Autodesk Inventor part; units mm, degrees
ref_plane "YZ Plane" through (0, 0, 0) normal (1, 0, 0) x (0, 1, 0)
ref_plane "XZ Plane" through (0, 0, 0) normal (0, 1, 0) x (-1, 0, 0)
ref_plane "XY Plane" through (0, 0, 0) normal (0, 0, 1) x (1, 0, 0)
sketch "Sketch1" plane through (0, 0, 0) normal (1, 0, 0) x (0, 1, 0)
  line L0 (0, 0) -> (2.5, 0)
  line L1 (0, 0) -> (4, 0)
  line L2 (2.5, 0) -> (2.5, -7)
  line L3 (2.5, -7) -> (0, -7)
  line L4 (0, -7) -> (20, -7)
  line L5 (4, 0) -> (4, -7)
  line L6 (2.5, -7) -> (2.5, -41)
  line L7 (20, -7) -> (20, -11)
  line L8 (20, -11) -> (2.5, -11)
  line L9 (20, -7) -> (22.5, -7)
  line L10 (22.5, -7) -> (22.5, -11)
  line L11 (22.5, -11) -> (20, -11)
  line L12 (20, -11) -> (20, -7)
  line L13 (20, -7) -> (20, -11)
  line L14 (4, 0) -> (2.5, 0)
  line L15 (2.5, 0) -> (2.5, -11)
  line L16 (2.5, -11) -> (4, -11)
  line L17 (4, -11) -> (4, 0)
  line L18 (2.5, -11) -> (22.5, -11)
  line L19 (22.5, -11) -> (22.5, -7)
  line L20 (22.5, -7) -> (2.5, -7)
  line L21 (2.5, -7) -> (2.5, -11)
  line L22 (2.5, -11) -> (6.5, -11)
  line L23 (0, -7) -> (0, -105.9451)
  line L24 (2.5, -41) -> (25, -41)
  line L25 (0, -82) -> (2.5, -82)
  line L26 (0, -82) -> (4, -82)
  line L27 (2.5, -82) -> (2.5, -75)
  line L28 (2.5, -75) -> (0, -75)
  line L29 (0, -75) -> (20, -75)
  line L30 (4, -82) -> (4, -75)
  line L31 (20, -75) -> (20, -71)
  line L32 (20, -71) -> (2.5, -71)
  line L33 (20, -75) -> (22.5, -75)
  line L34 (22.5, -75) -> (22.5, -71)
  line L35 (22.5, -71) -> (20, -71)
  line L36 (20, -71) -> (20, -75)
  line L37 (20, -75) -> (20, -71)
  line L38 (4, -82) -> (2.5, -82)
  line L39 (2.5, -82) -> (2.5, -71)
  line L40 (2.5, -71) -> (4, -71)
  line L41 (4, -71) -> (4, -82)
  line L42 (2.5, -71) -> (22.5, -71)
  line L43 (22.5, -71) -> (22.5, -75)
  line L44 (22.5, -75) -> (2.5, -75)
  line L45 (2.5, -75) -> (2.5, -71)
  line L46 (2.5, -71) -> (6.5, -71)
  line L47 (2.5, -11) -> (6.5, -11)
  line L48 (6.5, -11) -> (6.5, -71)
  line L49 (6.5, -71) -> (2.5, -71)
  line L50 (2.5, -71) -> (2.5, -11)
  line L51 (6.5, -11) -> (9.5, -11)
  line L52 (9.5, -11) -> (9.5, -14)
  line L53 (9.5, -14) -> (6.5, -14)
  line L54 (6.5, -14) -> (6.5, -11)
  line L55 (6.5, -71) -> (9.5, -71)
  line L56 (9.5, -71) -> (9.5, -68)
  line L57 (9.5, -68) -> (6.5, -68)
  line L58 (6.5, -68) -> (6.5, -71)
  dimension "d1" = 2.5
  dimension "d2" = 4
  dimension "d3" = 7
  dimension "d4" = 20
  dimension "d5" = 34
  dimension "d9" = 4
  dimension "d12" = 2.5
  dimension "d13" = 4
  dimension "d55" = 22.5
  dimension "d56" = 4
  dimension "d80" = 3
  dimension "d81" = 3
  dimension "d82" = 3
  dimension "d83" = 3
revolve "Revolution2" add sketch "Sketch1" angle 360 about axis through (0, 0, -7) along (0, 0, -1) contours L1 L5 L4 L2 | L4 L17 L8 L6 | L4 L7 L8 L17 | L8 L48 L24 L6 | L9 L10 L11 L7 | L24 L48 L32 L50 | L8 L52 L53 L48 | L29 L30 L26 L27 | L39 L32 L41 L29 | L41 L32 L31 L29 | L57 L56 L32 L48 | L31 L35 L34 L33
sketch "Sketch6" plane through (0, 0, 0) normal (0, 1, 0) x (-1, 0, 0)
  line L0 (-2.5, -82) -> (2.5, -82)
  line L1 (0, -82) -> (0, -62)
  line L2 (0, -82) -> (20, -82) construction
  line L3 (0, -65) -> (15, -65) construction
  line L4 (0, -59) -> (15, -59) construction
  line L5 (10.6066, -48.3934) -> (10.6066, -54.3934)
  line L6 (0, -65) -> (0, -59)
  line L7 (0, -62) -> (0, -59.5)
  line L8 (0, -59.5) -> (10.6066, -48.8934)
  line L9 (10.6066, -48.8934) -> (10.6066, -53.8934)
  line L10 (10.6066, -53.8934) -> (0, -64.5)
  line L11 (0, -59.5) -> (0, -64.5)
  point P0 (0, 0)
  dimension "d64" = 20
  dimension "d65" = 90
  dimension "d69" = 15
  dimension "d71" = 15
  dimension "d75" = 2.5
  dimension "d76" = 5
extrude "Extrusion6" cut sketch "Sketch6" along normal mid plane 5
sketch "Sketch7" plane through (0, 0, 0) normal (0, 0, 1) x (1, 0, 0)
  arc A0 (-1.9966, -1.5104) -> (-1.9966, 1.4896) centre (0.0034, -0.0104) ccw
  line L0 (-1.9966, -0.0104) -> (-1.9966, 1.4896)
  line L1 (-1.9966, -0.0104) -> (-1.9966, -1.5104)
  line L2 (-1.9966, 1.4896) -> (-1.9966, -2.007)
  line L3 (-1.9966, -2.007) -> (-3.9862, -2.007)
  line L4 (-3.9862, -2.007) -> (-3.9862, 1.4896)
  line L5 (-3.9862, 1.4896) -> (-1.9966, 1.4896)
  line L6 (-1.9966, -1.5104) -> (-3.2272, -1.5104)
  line L7 (-3.2272, -1.5104) -> (-3.2272, 1.4896)
  line L8 (-3.2272, 1.4896) -> (-1.9966, 1.4896)
  line L9 (-1.9966, 1.4896) -> (-1.9966, -1.5104)
  point P0 (0, 0)
  point P1 (0, 0)
  dimension "d77" = 5
extrude "Extrusion7" add sketch "Sketch7" against normal blind 26 contours L6 L7 L5 L0 L1
sketch "Sketch11" plane through (0, 0, -71) normal (0, 0, 1) x (1, 0, 0)
  circle A0 centre (0, 0) radius 2.5
  circle A1 centre (0, 0) radius 9.5
  arc A2 (0, 2.5) -> (0, -2.5) centre (0, 0) ccw
  circle A3 centre (0, 0) radius 46.837
  point P0 (0, 0)
  dimension "d90" = 19
extrude "Extrusion11" cut sketch "Sketch11" against normal blind 100 contours A0 | A1 | A3
sketch "Sketch12" plane through (0, 0, -71) normal (0, 0, -1) x (-1, 0, 0)
  circle A0 centre (0, 0) radius 9.5
  circle A1 centre (0, 0) radius 9.5
  circle A2 centre (0, 0) radius 6.5
  point P0 (0, 0)
extrude "Extrusion12" add sketch "Sketch12" along normal blind 2
sketch "Sketch13" plane through (0, 0, -11) normal (0, 0, -1) x (-1, 0, 0)
  circle A0 centre (0, 0) radius 46.586
extrude "Extrusion13" cut sketch "Sketch13" against normal blind 30
sketch "Sketch14" plane through (0, 0, -11) normal (0, 0, 1) x (1, 0, 0)
  circle A0 centre (0, 0) radius 9.5
  circle A1 centre (0, 0) radius 9.5
  arc A2 (0, 2.5) -> (0, -2.5) centre (0, 0) ccw
  circle A3 centre (0, 0) radius 6.5
  dimension "d97" = 19
  dimension "d98" = 13
extrude "Extrusion14" add sketch "Sketch14" along normal blind 2
properties part number "Spool_revB3"
Read the model definition and answer for the solid it produces. Units are mm, in the model's axes. A direction names the side the tool comes from. Coordinates: 2 decimals unless noted, no trailing zeros. Write each loop counter-clockwise with the first axis right and the second up, starting at its lowest first coordinate (ties: lowest second). Pieces come first, ordered by that corner, then holes. Notation, with made-up numbers: M -38,-25 L -3,-25 A33 cw -3,14 Z; hole C 27,87 d3. An arc over 180 degrees is marked long. Use a Markdown table: item, result.
Q1. The part is cut by section A-A, the plane y = -7.5. Write down the section's boundary in (x, z).
Answer block:
| item | result |
|---|---|
| outline | M -5.83,-73 L 5.83,-73 L 5.83,-68 L -5.83,-68 Z; M -5.83,-14 L 5.83,-14 L 5.83,-9 L -5.83,-9 Z |
Q2. Straight lines are drawn through the part: L1, parallel to Y at x = -0.25, z = -26; L2, parallel to Z at x = -6.75, y = 6.5; L3, parallel to Y at x = 0, z = -10.6. For each, find the intervals that lie inside material, in ascending order. Write a range as [from, to].
Answer block:
| item | result |
|---|---|
| L1 | y = [-6.5, -2.49], [2.49, 6.5] |
| L2 | z = [-73, -68], [-14, -9] |
| L3 | y = [-9.5, -6.5], [6.5, 9.5] |
Q3. The part is cut by section B-B, the plane z = -29. Write down the section's boundary in (x, y), then the cut area to 3 significant figures.
Answer block:
| item | result |
|---|---|
| outline | C 0,0 d13; hole C 0,0 d5 |
| area | 113 mm2 |
Q4. Each of these flat-tipped pins is pushed along its axis until it touches: pin 1 Ø3 at (x, y) = (0, 0) entering from +Z; pin 2 Ø6 at (x, y) = (4.5, -0.5) entering from +Z; pin 3 Ø5 at (x, z) = (-7, -41.5) entering from +Y; pin 4 Ø3 at (y, z) = (5.5, -57.5) entering from +X. Where does it stop, or does it pass through?
Answer block:
| item | result |
|---|---|
| pin 1 | passes through |
| pin 2 | stops at z = -9 |
| pin 3 | stops at y = 4.69 |
| pin 4 | stops at x = 5.12 |
Q5. Determine the mould class of faces 1 (the face through (-3, -2.5, -59)), 2 (the face through (-5.158, 3.955, -10.014)), 3 (the face through (6.445, -0.846, -41.378)), 4 (the face through (-6, 4, -68)) for opening direction X: released by +X, released by -X, zero draft, split by the parting line, or undercut.
Answer block:
| item | result |
|---|---|
| face 1 | undercut |
| face 2 | undercut |
| face 3 | split by the parting line |
| face 4 | zero draft |
Q6. Which of the six approach directions +Z, -Z, +X, -X, +Y, -Y give full straight-line access (tool end or side, diameter ignored) to faces 5 (the face through (-4, 0, -60.5)), 6 (the face through (-1.997, 0, -18)), 7 (the face through (-3, 0, -11)), 8 (the face through (5.158, 3.955, -71.986))?
Answer block:
| item | result |
|---|---|
| face 5 | none |
| face 6 | +Z, -Z |
| face 7 | +Z |
| face 8 | -Z |
